CAD build for the part. Positions are in the model's coordinates, mm. A direction names the side the tool comes from. Give positions to 0.01 mm unless a question says otherwise; leave off trailing zeros. Write each loop counter-clockwise with the first axis right and the second up, starting at its lowest first coordinate (ties: lowest second). Pieces come first, ordered by that corner, then holes. Notation, with made-up numbers: (-13.5, 36.5) -> (28.5, 36.5) arc R24 ccw to (28.5, 61.5) -> close; hole circle Ø6 at (6, 40.25). An arc over 180 degrees is marked (long way). Answer in a Markdown table with one row per item. Add a question column.
```python
from build123d import *

# Parameters (mm, degrees)
SKETCH_1_R          = 11.25
EXTRUDE_1_DEPTH     = 11
SKETCH_2_R          = 1.15
CUT_EXTRUDE_1_DEPTH = 20.342311134
SKETCH_4_W          = 7
SKETCH_4_H          = 7
EXTRUDE_3_DEPTH     = 6
SKETCH_5_R          = 2.05
CUT_EXTRUDE_2_DEPTH = 9.5
FILLET_1_R          = 1


with BuildPart() as part:
    # 草图1 → 凸台-拉伸1 (new body)
    with BuildSketch(Plane(origin=(0, 0, 0), x_dir=(1, 0, 0), z_dir=(0, 1, 0))):
        with Locations(Location((0, 0, 0), (0, 0, 270))):
            Circle(SKETCH_1_R)
    extrude(amount=EXTRUDE_1_DEPTH)

    # 草图2 → 切除-拉伸1 (cut, through all)
    with BuildSketch(Plane.XZ):
        with Locations(Location((8.5, 0, 0), (0, 0, 270))):
            Circle(SKETCH_2_R)
        with Locations(Location((-8.5, 0, 0), (0, 0, 90))):
            Circle(SKETCH_2_R)
    extrude(amount=-CUT_EXTRUDE_1_DEPTH, mode=Mode.SUBTRACT)

    # 草图4 → 凸台-拉伸3 (add)
    with BuildSketch(Plane(origin=(0, 11, 0), x_dir=(1, 0, 0), z_dir=(0, 1, 0))):
        Rectangle(SKETCH_4_W, SKETCH_4_H)
    extrude(amount=EXTRUDE_3_DEPTH)

    # 草图5 → 切除-拉伸2 (cut)
    with BuildSketch(Plane(origin=(0, 11, 0), x_dir=(1, 0, 0), z_dir=(0, 1, 0))):
        with Locations(Location((8.5, 0, 0), (0, 0, 270))):
            Circle(SKETCH_5_R)
        with Locations(Location((-8.5, 0, 0), (0, 0, 270))):
            Circle(SKETCH_5_R)
    extrude(amount=-CUT_EXTRUDE_2_DEPTH, mode=Mode.SUBTRACT)

    # 圆角1
    fillet_1_edges = [part.edges().sort_by_distance(p)[0] for p in [
        (3.5, 14, 3.5),
        (3.5, 14, -3.5),
        (-3.5, 14, -3.5),
        (-3.5, 14, 3.5),
    ]]
    fillet(fillet_1_edges, radius=FILLET_1_R)


solid = part.part
```
Item 1: Which spindle directions (+Z, -Z, +X, -X, +Y, -Y) get a long thin tool onto all of the face, cutting with end or side? Do faces 1 (the face through (0, 14, -3.5)), 2 (the face through (-8.5, 1.5, 1.3)), 3 (the face through (3.199, 14.042, 3.215)), 4 (the face through (0, 14, 3.5)), 5 (the face through (-3.215, 14.042, -3.199)). Say none if no direction does.
Item 2: Drop flat-ended pins along their axis: pin 1 Ø10 at (x, z) = (-9, 0) entering from +Y; pin 2 Ø3.5 at (x, z) = (-8.5, 0) entering from +Y; pin 3 Ø8 at (y, z) = (3.5, 4.5) entering from -X. Give the stop position or say it passes through.
Item 3: Slice it at D-D, the plane x = -8.5. List the corners of the cut face in (y, z), then the cut area to 3 significant figures.
Item 4: Slice it at B-B, the plane x = 0. List the corners of the cut face in (y, z), then the cut area to 4 significant figures.
Item 5: Probe L1, parallel to X at y = 0.55, z = 0; L2, parallel to X at y = 9, z = 0; L3, parallel to Y at x = -7.25, z = -3.5. List the from-to ranges inside material, lowest first. Write a range as from..to.
Item 6: Slice it at C-C, the plane y = 13. List the corners of the cut face in (x, z), then the cut area to 3 significant figures.
Item 7: Slice it at A-A, the plane z = 0. List the corners of the cut face in (x, y), then the cut area to 3 significant figures.
Item 8: Mould opens along X. For faces 6 (the face through (-4.31, 5.42, 10.39)), 7 (the face through (-3.5, 14, 0)), 8 (the face through (3.215, 14.042, -3.199)), 9 (the face through (7, 1.5, 0)) say: released by +X, released by -X, zero draft, split by the parting line, or undercut.
Answer key:
| question | item | result |
|---|---|---|
| 1 | face 1 | -Z, +X, -X, +Y |
| 1 | face 2 | +Y |
| 1 | face 3 | +Z, +X, +Y |
| 1 | face 4 | +Z, +X, -X, +Y |
| 1 | face 5 | -Z, -X, +Y |
| 2 | pin 1 | stops at y = 11 |
| 2 | pin 2 | stops at y = 1.5 |
| 2 | pin 3 | stops at x = -11.24 |
| 3 | outline | (0, -7.37) -> (11, -7.37) -> (11, -2.05) -> (1.5, -2.05) -> (1.5, -1.15) -> (0, -1.15) -> close; (0, 1.15) -> (1.5, 1.15) -> (1.5, 2.05) -> (11, 2.05) -> (11, 7.37) -> (0, 7.37) -> close |
| 3 | area | 120 mm² |
| 4 | outline | (0, -11.25) -> (11, -11.25) -> (11, -3.5) -> (17, -3.5) -> (17, 3.5) -> (11, 3.5) -> (11, 11.25) -> (0, 11.25) -> close |
| 4 | area | 289.5 mm² |
| 5 | L1 | x = -11.25..-9.65, -7.35..7.35, 9.65..11.25 |
| 5 | L2 | x = -11.25..-10.55, -6.45..6.45, 10.55..11.25 |
| 5 | L3 | y = 0..11 |
| 6 | outline | (-3.5, -2.5) arc R1 ccw to (-2.5, -3.5) -> (2.5, -3.5) arc R1 ccw to (3.5, -2.5) -> (3.5, 2.5) arc R1 ccw to (2.5, 3.5) -> (-2.5, 3.5) arc R1 ccw to (-3.5, 2.5) -> close |
| 6 | area | 48.1 mm² |
| 7 | outline | (-11.25, 0) -> (-9.65, 0) -> (-9.65, 1.5) -> (-10.55, 1.5) -> (-10.55, 11) -> (-11.25, 11) -> close; (-7.35, 0) -> (7.35, 0) -> (7.35, 1.5) -> (6.45, 1.5) -> (6.45, 11) -> (3.5, 11) -> (3.5, 17) -> (-3.5, 17) -> (-3.5, 11) -> (-6.45, 11) -> (-6.45, 1.5) -> (-7.35, 1.5) -> close; (9.65, 0) -> (11.25, 0) -> (11.25, 11) -> (10.55, 11) -> (10.55, 1.5) -> (9.65, 1.5) -> close |
| 7 | area | 205 mm² |
| 8 | face 6 | split by the parting line |
| 8 | face 7 | released by -X |
| 8 | face 8 | released by +X |
| 8 | face 9 | undercut |
